Read the model definition and answer for the solid it produces. Units are mm, in the model's axes. Coordinates: 2 decimals unless noted, no trailing zeros. Write each loop counter-clockwise with the first axis right and the second up, starting at its lowest first coordinate (ties: lowest second). Pieces come first, ordered by that corner, then holes. Notation, with made-up numbers: (38.5, 58.25) -> (76.5, 58.25) arc R20 ccw to (76.5, 80.25) -> close; hole circle Ø2 at (67.25, 23). An arc over 180 degrees is marked (long way). Answer as a JSON object with one key per item and string values. Group by question number.
(1) Find section A-A (y = 0). Give the vertices of the cut face in (x, z).
(2) Find section C-C (z = 17). Give the vertices of the cut face in (x, y).
(3) Flat-ended cylindrical pins translate along their axes: P1, Ø1, axis at x = 2, z = 34, coming from the +Y side; P2, Ø3, axis at x = -3.5, z = 71, coming from the +Y side; P3, Ø1.5, axis at y = 7.5, z = 105.5, coming from the -X side. Find the tip coordinate at first contact, or state that the pin passes through.
(4) Straight lines are drawn through the part: L1, parallel to X at y = 0, z = 76.5; L2, parallel to Y at x = 6, z = 187.5. For each, find the intervals that lie inside material, in ascending order.
(5) Find section B-B (x = 0). Give the vertices of the cut face in (y, z).
Autodesk Inventor part; units mm, degrees
ref_plane "Start Plane" through (0, 0, -2.5789) normal (0, 0, 1) x (1, 0, 0)
ref_plane "End Plane" through (0, 0, 212.6682) normal (0, 0, 1) x (1, 0, 0)
ref_plane "Work Plane4" through (-10.6194, 1.0174, -13.521) normal (0.7815, -0.0749, -0.6194) x (-0.6047, 0.1537, -0.7815)
ref_plane "Start Plane" through (0, 0, -2.5789) normal (0, 0, 1) x (1, 0, 0)
ref_plane "End Plane" through (0, 0, 212.6682) normal (0, 0, 1) x (1, 0, 0)
sketch "Sketch" plane through (0, 0, 0) normal (0, 0, 1) x (1, 0, 0)
  circle A0 centre (0, 0) radius 6.9342
  circle A1 centre (0, 0) radius 10.668
  dimension "d0" = 21.336
  dimension "d1" = 3.7338
extrude "Body" add sketch "Sketch" along normal up to surface (215.2472 mm away) from surface at -2.5789
sketch "Sketch3" plane through (0, 0, 0) normal (0, 0, 1) x (1, 0, 0)
  line L0 (0, 0) -> (10, 0)
ref_plane "Work Plane3" through (0, 0, 0) normal (0, -1, 0) x (1, 0, 0)
sketch "Sketch4" plane through (0, 0, 0) normal (0, -1, 0) x (1, 0, 0)
  line L0 (-2, -2.5789) -> (12, -2.5789)
  line L1 (-2, 212.6682) -> (12, 212.6682)
  dimension "d7" = 215.2472
ref_plane "Work Plane4" through (-10.6194, 1.0174, -13.521) normal (0.7815, -0.0749, -0.6194) x (-0.6047, 0.1537, -0.7815)
split "Split1" plane through (-10.6194, 1.0174, -13.521) removes the side toward (0.7815, -0.0749, -0.6194)
ref_plane "Work Plane5" through (8.9776, -5.7627, -9.228) normal (-0.5506, 0.3534, -0.7563) x (-0.2438, 0.7984, 0.5506)
split "Split2" plane through (8.9776, -5.7627, -9.228) removes the side toward (-0.5506, 0.3534, -0.7563)
ref_plane "Work Plane6" through (6.6005, -8.3809, 217.9879) normal (-0.4276, 0.543, 0.7227) x (0.8938, 0.1348, 0.4276)
split "Split3" plane through (6.6005, -8.3809, 217.9879) removes the side toward (-0.4276, 0.543, 0.7227)
ref_plane "Work Plane7" through (2.6801, -10.3259, 213.4307) normal (-0.1175, 0.4527, 0.8839) x (0.9927, 0.0282, 0.1175)
split "Split4" plane through (2.6801, -10.3259, 213.4307) removes the side toward (-0.1175, 0.4527, 0.8839)
ref_plane "Work Plane8" through (-10.0134, -3.6794, 216.1428) normal (0.5789, 0.2127, 0.7872) x (0.8125, -0.0689, -0.5789)
split "Split5" plane through (-10.0134, -3.6794, 216.1428) removes the side toward (0.5789, 0.2127, 0.7872)
equation "\"d0\" = G_H"
equation "\"d1\" = G_T"
equation "\"d2\" = G_L"
equation "\"G_H\" = 21.336"
equation "\"G_T\" = 3.7338"
equation "\"G_L\" = 215.24716"
equation "\"G_OFFSET_START\" = 2.57893"
equation "\"G_OFFSET_END\" = 4.88279"
equation "\"d4\" = -G_OFFSET_START"
equation "\"d5\" = G_OFFSET_END + B_L"
equation "\"B_L\" = 207.78544"
properties part number "ANSI - 1/2 x 0.147 - 8.474" material "Steel, Mild"
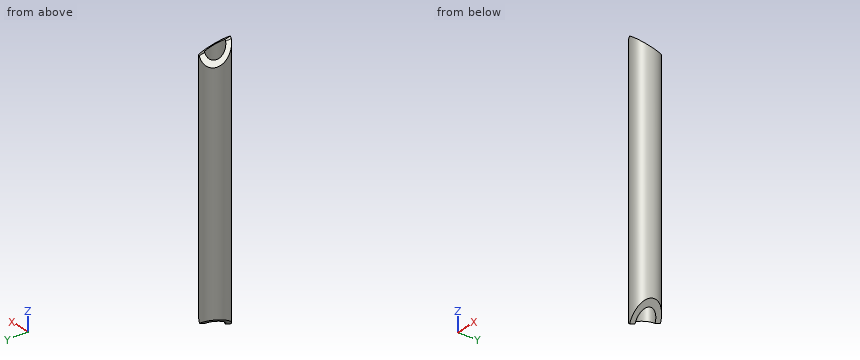
Results below:
{
 "1": {"outline": "(-10.67, 7.77) -> (-6.93, 5.05) -> (-6.93, 203.68) -> (-10.67, 201.47) -> close; (6.93, 8.75) -> (10.67, 13.46) -> (10.67, 199.94) -> (6.93, 202.69) -> close"},
 "2": {"outline": "circle Ø21.34 at (0, 0); hole circle Ø13.87 at (0, 0)"},
 "3": {"P1": "stops at y = 10.56", "P2": "stops at y = 10.48", "P3": "stops at x = -8.26"},
 "4": {"L1": "x = -10.67 to -6.93, 6.93 to 10.67", "L2": "y = -8.82 to -3.48, 3.48 to 8.82"},
 "5": {"outline": "(-10.67, 1.29) -> (-6.93, 0.84) -> (-6.93, 209.66) -> (-10.67, 210.67) -> close; (6.93, 3.24) -> (10.67, 4.99) -> (10.67, 199.77) -> (6.93, 202.58) -> close"}
}
